Can you work these out from the model? Positions are in its coordinate system, mm. Give positions to 0.01 mm unless a question says otherwise; leave off trailing zeros. Loops run counter-clockwise (first coordinate to the right, second up) from the corner with the lowest first, then second, coordinate; pieces in that order, holes last. Notation, with made-up numbers: M 52,11 L 76,11 A14 cw 76,18 Z; hole C 7.25,49.25 d9. An arc over 180 degrees is marked long. Put each result on its own line as item: value. Start each with the question number.
1) Imagine slicing it at A-A (y = -43.5). Write out the boundary of the cut face in (x, z), then the cut area to 3 significant figures.
2) Please list where these lines run through material, in increasing order: line 1 along Z through (x, y) = (16, 11.5); line 2 along Y through (x, z) = (-22, 49.5); line 3 along Z through (x, y) = (16, -8). Write a range as from..to.
3) For P1, Ø8, axis at x = 33, y = 25, coming from the +Z side; P2, Ø3, axis at x = -31.5, z = 48.5, coming from the +Y side; P3, Ø3, axis at x = -53.5, y = 4.5, coming from the +Z side, each with a flat end and sliding along its axis, tell me the tip position at first contact or that it passes through.
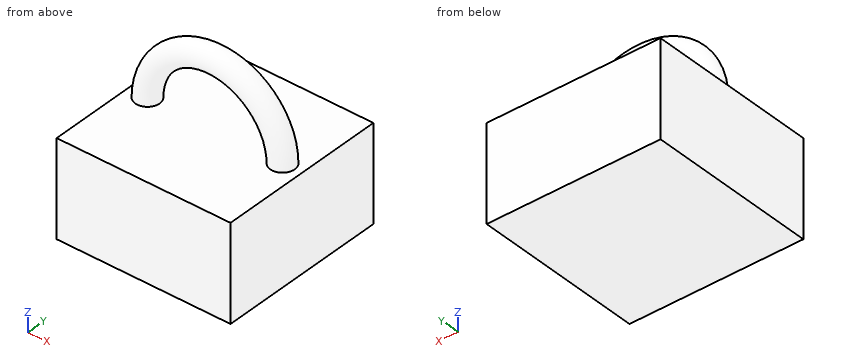
from build123d import *

# Parameters (mm, degrees)
F1_R     = 9.824635
F0_W     = 69.863096
F0_H     = 137.526572
F3_DEPTH = 76.8858


with BuildPart() as f2:
    # F1 (on Top) → F2 (revolve)
    with BuildSketch(Plane.XY):
        with Locations((54.264009, 0)):
            Circle(F1_R)
    revolve(axis=Axis((0, 0, 0), (0, -1, 0)))

    # F0 (on Top) → F3 (join)
    with BuildSketch(Plane.XY):
        with Locations((34.931548, 0)):
            Rectangle(F0_W, F0_H)
        with Locations((-34.931548, 0)):
            Rectangle(F0_W, F0_H)
    extrude(amount=-F3_DEPTH)


solid = f2.part
Recorded:
1. outline: M -69.86,-76.89 L 69.86,-76.89 L 69.86,0 L -69.86,0 Z
1. area: 10,700 mm²
2. line 1: -76.89..0
2. line 2: -9.82..9.82
2. line 3: -76.89..0, 45.85..57.79
3. P1: z = 0
3. P2: y = 9.6
3. P3: z = 35.89
